Can you work these out from the model? Positions are in its coordinate system, mm. Face numbers are marked on the shaded views. A direction names the side the tool comes from. Coordinates: 2 decimals unless noted, no trailing zeros. Loops run counter-clockwise (first coordinate to the right, second up) from the corner with the lowest first, then second, coordinate; pieces in that order, holes last. Notation, with made-up numbers: (80, 39.5) -> (135, 39.5) arc R32 cw to (135, 67.5) -> close; hole circle Ø9 at (-34.5, -5). An arc over 180 degrees is marked (long way). Use one line per item in the form item = value. Start each with the question number.
(1) On a 3-axis mill with a long thin cutter (end or side, diameter ignored), from which of +Z, -Z, +X, -X, +Y, -Y can I reach the whole of each face in a straight line? I mean the marked faces 1 and 2. Say none if no direction works.
(2) Imagine slicing it at C-C (z = 0). List the corners of the cut face in (x, y) for me (1 decimal), plus the area to 3 significant figures.
(3) Imagine slicing it at A-A (x = 5.5). List the corners of the cut face in (y, z) for me (1 decimal).
(4) Imagine slicing it at D-D (y = -86.5). List the corners of the cut face in (x, z) for me (3 decimals).
(5) I need wall thicknesses on line 1 (Y direction, x = 4, z = 7.5); line 2 (X direction, y = -52, z = 0.25); line 3 (Z direction, x = -0.5, y = -28.5). Which ranges of each line are inside material? Lowest first, please. Write a range as [from, to].
(6) Thinking about a two-plate mould opening in Y: for the marked faces 3, 4 and 5, which applies, released by +Y, released by -Y, zero draft, split by the parting line, or undercut?
(7) I'm going to push flat-ended pins straight in: pin 1 (2 mm diameter, centred on x = 2.5, y = -132, fed in from +Z); pin 2 (10 mm diameter, centred on x = 6, y = -14.5, fed in from +Z); pin 3 (4 mm diameter, centred on y = -123, z = 4.5, fed in from -X). Where does each tip first touch, or does it pass through?
(8) Imagine slicing it at B-B (z = -7). List the corners of the cut face in (x, y) for me (1 decimal), plus the area to 3 significant figures.
```python
from build123d import *

# Parameters (mm, degrees)
F0_R     = 3.175
F1_DEPTH = 136.5504
F2_W     = 19.05
F2_H     = 19.05
F3_DEPTH = 4.7625
F4_W     = 19.05
F4_H     = 19.05
F5_DEPTH = 4.7625
F6_R     = 3.175
F7_DEPTH = 25.4
F8_R     = 3.175
F9_DEPTH = 25.4


with BuildPart() as f1:
    # F0 (on Front) → F1 (new body)
    with BuildSketch(Plane.XZ):
        Circle(F0_R)
    extrude(amount=F1_DEPTH)

    # F2 (on face) → F3 (join)
    with BuildSketch(Plane.XZ.offset(136.5504)):
        Rectangle(F2_W, F2_H)
    extrude(amount=F3_DEPTH)

    # F4 (on face) → F5 (join)
    with BuildSketch(Plane(origin=(0, 0, 0), x_dir=(-1, 0, 0), z_dir=(0, 1, 0))):
        Rectangle(F4_W, F4_H)
    extrude(amount=F5_DEPTH)

    # F6 (on face) → F7 (join)
    with BuildSketch(Plane.XZ.offset(136.5504)):
        Circle(F6_R)
    extrude(amount=F7_DEPTH)

    # F8 (on face) → F9 (join)
    with BuildSketch(Plane(origin=(0, 0, 0), x_dir=(-1, 0, 0), z_dir=(0, 1, 0))):
        Circle(F8_R)
    extrude(amount=F9_DEPTH)


solid = f1.part
```
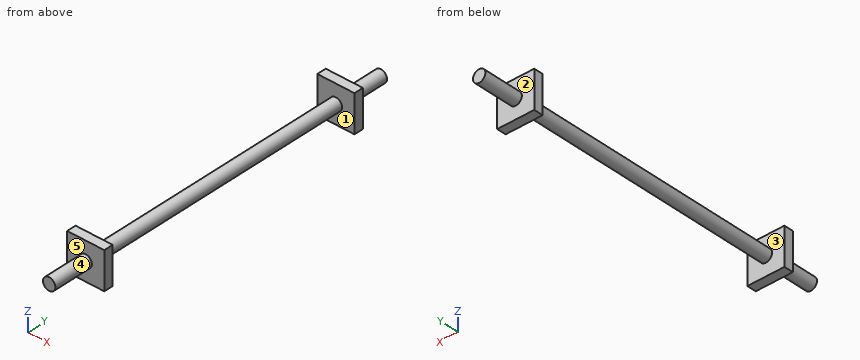
Worked out:
q1.face_1 = none
q1.face_2 = +Y
q2.outline = (-9.5, -141.3) -> (-3.2, -141.3) -> (-3.2, -162) -> (3.2, -162) -> (3.2, -141.3) -> (9.5, -141.3) -> (9.5, -136.6) -> (3.2, -136.6) -> (3.2, 0) -> (9.5, 0) -> (9.5, 4.8) -> (3.2, 4.8) -> (3.2, 25.4) -> (-3.2, 25.4) -> (-3.2, 4.8) -> (-9.5, 4.8) -> (-9.5, 0) -> (-3.2, 0) -> (-3.2, -136.6) -> (-9.5, -136.6) -> close
q2.area = 1,310 mm2
q3.outline = (-141.3, -9.5) -> (-136.6, -9.5) -> (-136.6, 9.5) -> (-141.3, 9.5) -> close; (0, -9.5) -> (4.8, -9.5) -> (4.8, 9.5) -> (0, 9.5) -> close
q4.outline = circle Ø6.35 at (0, 0)
q5.line_1 = [-141.31, -136.55], [0, 4.76]
q5.line_2 = [-3.17, 3.17]
q5.line_3 = [-3.14, 3.14]
q6.face_3 = undercut
q6.face_4 = zero draft
q6.face_5 = released by -Y
q7.pin_1 = 2.8
q7.pin_2 = 3.01
q7.pin_3 = -1.96
q8.outline = (-9.5, -141.3) -> (9.5, -141.3) -> (9.5, -136.6) -> (-9.5, -136.6) -> close; (-9.5, 0) -> (9.5, 0) -> (9.5, 4.8) -> (-9.5, 4.8) -> close
q8.area = 181 mm2
